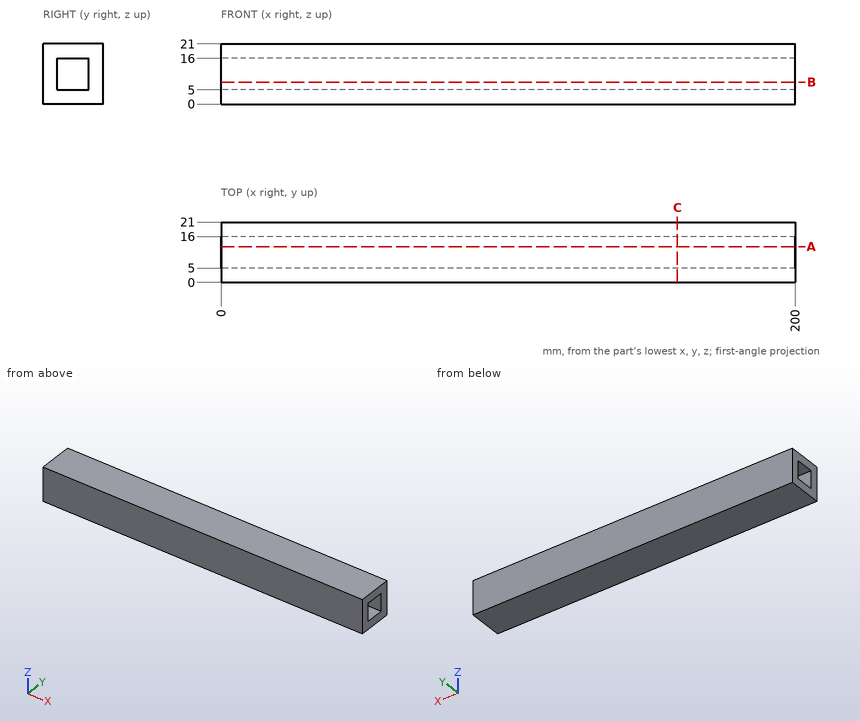
Study the drawing (mm; zero at the part's minimum x, y, z) and answer. Coordinates: 2 decimals unless noted, no trailing zeros. Write each loop counter-clockwise with the first axis right and the second up, starting at its lowest first coordinate (ties: lowest second). Pieces come first, ordered by that corner, then holes. Notation, with made-up numbers: M 33,-31.5 L 58,-31.5 A9 ccw 58,-20.5 Z; hole C 42.5,-8.5 d4. An arc over 180 degrees is marked long. Use a Markdown table: item, result. Add a question column.
1. Section A-A (y = 12.5) is taken. Give the vertices of the cut face in (x, z).
2. Section C-C (x = 159) is taken. Give the vertices of the cut face in (y, z).
3. Given P1, Ø3.5, axis at x = 108, z = 8, coming from the -Y side, flat-ended and moving along its own axis, determine where the tip first touches the part or whether it passes through.
4. A straight line is drawn through the part: line 1 along Y through (x, z) = (34.5, 11). Find the intervals that lie inside material, in ascending order. Write a range as [from, to].
Data:
| question | item | result |
|---|---|---|
| 1 | outline | M 0,0 L 200,0 L 200,5 L 0,5 Z; M 0,16 L 200,16 L 200,21 L 0,21 Z |
| 2 | outline | M 0,0 L 21,0 L 21,21 L 0,21 Z; hole M 5,5 L 16,5 L 16,16 L 5,16 Z |
| 3 | P1 | stops at y = 0 |
| 4 | line 1 | y = [0, 5], [16, 21] |
